```python
from build123d import *

# Parameters (mm, degrees)
F0_W     = 17.519105383
F0_H     = 17.8348239851
F0_R     = 2.0418919941
F1_DEPTH = 60
F2_DEPTH = 64


with BuildPart() as f1:
    # F0 (on Top) → F1 (new body)
    with BuildSketch(Plane.XY):
        with BuildLine():
            Line((-8.7595526915, 8.9174119926), (8.7595526915, 8.9174119926))
            ThreePointArc((8.7595526915, 8.9174119926), (0, 12.5), (-8.7595526915, 8.9174119926))
        make_face()
        with BuildLine():
            Line((-8.7595526915, -8.9174119926), (-8.7595526915, 8.9174119926))
            ThreePointArc((-8.7595526915, 8.9174119926), (-12.5, 0), (-8.7595526915, -8.9174119926))
        make_face()
        with BuildLine():
            ThreePointArc((-8.7595526915, -8.9174119926), (0, -12.5), (8.7595526915, -8.9174119926))
            Line((8.7595526915, -8.9174119926), (-8.7595526915, -8.9174119926))
        make_face()
        with BuildLine():
            ThreePointArc((8.7595526915, -8.9174119926), (11.5270206177, -4.835059015), (12.5, 0))
            ThreePointArc((12.5, 0), (11.5270206177, 4.835059015), (8.7595526915, 8.9174119926))
            Line((8.7595526915, 8.9174119926), (8.7595526915, -8.9174119926))
        make_face()
        Rectangle(F0_W, F0_H)
        Circle(F0_R, mode=Mode.SUBTRACT)
    extrude(amount=F1_DEPTH)

    # F0 (on Top) → F2 (join)
    with BuildSketch(Plane.XY):
        Circle(F0_R)
    extrude(amount=F2_DEPTH)


solid = f1.part
```
Can you work these out from the model? Positions are in its coordinate system, mm. A direction names the side the tool comes from. Coordinates: 2 decimals unless noted, no trailing zeros. Order: outer loops, then holes, each group sorted by start corner. A loop starts at its lowest first (then second) coordinate and runs counter-clockwise, first axis right, second up. Notation, with made-up numbers: (1.25, 77.25) -> (5.25, 77.25) arc R20 cw to (5.25, 95.25) -> close; hole circle Ø2 at (-15.5, -2). An arc over 180 degrees is marked (long way). Write each question's results on one line, items separated by ' | '.
Item 1: I want a section at B-B, the plane z = 46.5. Write out the boundary of the cut face in (x, y).
Results are:
outline: circle Ø25 at (0, 0)
Item 2: I'm going to push flat-ended pins straight in: pin 1 Ø1.5 at (y, z) = (2, 37) entering from +X; pin 2 Ø4 at (x, z) = (6, 47) entering from +Y; pin 3 Ø4 at (x, z) = (7, 30) entering from +Y. Where does each tip first touch, or does it pass through?
Results are:
pin 1: x = 12.44 | pin 2: y = 11.84 | pin 3: y = 11.46
Item 3: Which directions (+Z, -Z, +X, -X, +Y, -Y) give clear straight access to the entire face, cutting with the end or side of a thin tool? Please do faces 1 (the face through (0, 0, 64)), 2 (the face through (1.95, 0.61, 61.97)).
Results are:
face 1: +Z, +X, -X, +Y, -Y | face 2: +Z
Item 4: I want a section at C-C, the plane y = 7.5. Write out the boundary of the cut face in (x, z).
Results are:
outline: (-10, 0) -> (10, 0) -> (10, 60) -> (-10, 60) -> close
Item 5: If I drill on line 1 along Z through (x, y) = (8.25, -5.5); line 2 along Y through (x, z) = (-0.5, 32); line 3 along Y through (x, z) = (8.75, 59), over which ranges is the centre line in solid material (lowest first)?
Results are:
line 1: 0 to 60 | line 2: -12.49 to 12.49 | line 3: -8.93 to 8.93
Item 6: I want a section at A-A, the plane x = 0. Write out the boundary of the cut face in (y, z).
Results are:
outline: (-12.5, 0) -> (12.5, 0) -> (12.5, 60) -> (2.04, 60) -> (2.04, 64) -> (-2.04, 64) -> (-2.04, 60) -> (-12.5, 60) -> close
